```python
from build123d import *

# Parameters (mm, degrees)
SKETCH2_R               = 1
BOSS_EXTRUDE2_DEPTH     = 10
SKETCH4_R               = 3.5
BOSS_EXTRUDE3_DEPTH     = 10
CHAMFER1_SIZE           = 5.282754963
CHAMFER1_SIZE_2         = 3.05
CUT_EXTRUDE4_DEPTH      = 21.603397778
CUT_EXTRUDE4_DEPTH_BACK = 21.603397778
SKETCH5_R               = 1
SKETCH6_R               = 1.5
BOSS_EXTRUDE4_DEPTH     = 1
SKETCH7_R               = 2
BOSS_EXTRUDE5_DEPTH     = 4
CHAMFER2_SIZE           = 0.5


# Some blends are built 0.0001 mm under size
with BuildPart() as part:
    # Sketch1 → Revolve1 (revolve)
    with BuildSketch(Plane.XY):
        with BuildLine():
            Line((0, 0), (0, -2))
            ThreePointArc((0, -2), (2, 0), (0, 2))
            Line((0, 2), (0, 0))
        make_face()
    revolve(axis=Axis((0, 0, 0), (0, 1, 0)))

    # Sketch2 → Boss-Extrude2 (add)
    with BuildSketch(Plane(origin=(0, 0, 0), x_dir=(1, 0, 0), z_dir=(0, 1, 0))):
        with Locations(Location((0, 0, 0), (0, 0, 90))):
            Circle(SKETCH2_R)
    extrude(amount=BOSS_EXTRUDE2_DEPTH)

    # Sketch4 → Boss-Extrude3 (add)
    with BuildSketch(Plane(origin=(0, 10, 0), x_dir=(1, 0, 0), z_dir=(0, 1, 0))):
        with Locations(Location((0, 0, 0), (0, 0, 270))):
            Circle(SKETCH4_R)
    extrude(amount=BOSS_EXTRUDE3_DEPTH)

    # Chamfer1
    # the kernel refuses this chamfer: 5.282754963, 3.05 mm, written as the material it takes off along each edge
    with BuildSketch(Plane(origin=(0, 10, 0), x_dir=(0, 0, 1), z_dir=(-1, 0, 0))) as chamfer1_piece_1_section:
        Polygon((3.5, CHAMFER1_SIZE), (3.5 - CHAMFER1_SIZE_2, 0), (3.5, 0), align=None)
    chamfer1_piece_1 = revolve(axis=Axis((0, 10, 0), (0, 1, 0)), mode=Mode.PRIVATE)
    chamfer1_piece_1 = chamfer1_piece_1 - Plane(origin=(0, 13.183046822, 0), x_dir=(0, 0, -1), z_dir=(0, -1, 0)) * Cylinder(1, 22, mode=Mode.PRIVATE)
    add(chamfer1_piece_1, mode=Mode.SUBTRACT)

    # Sketch5 → Cut-Extrude4 (cut, two sides: drawn at the far end of the back side and taken through both)
    with BuildSketch(Plane(origin=(0, 0, 0), x_dir=(0, 0, -1), z_dir=(1, 0, 0)).offset(-CUT_EXTRUDE4_DEPTH_BACK)):
        with Locations((0, 17.641377482)):
            Circle(SKETCH5_R)
    extrude(amount=CUT_EXTRUDE4_DEPTH + CUT_EXTRUDE4_DEPTH_BACK, mode=Mode.SUBTRACT)

    # Sketch6 → Boss-Extrude4 (add)
    with BuildSketch(Plane(origin=(0, 20, 0), x_dir=(1, 0, 0), z_dir=(0, 1, 0))):
        with Locations(Location((0, 0, 0), (0, 0, 270))):
            Circle(SKETCH6_R)
    extrude(amount=BOSS_EXTRUDE4_DEPTH)

    # Sketch7 → Boss-Extrude5 (add)
    with BuildSketch(Plane(origin=(0, 21, 0), x_dir=(1, 0, 0), z_dir=(0, 1, 0))):
        with Locations(Location((0, 0, 0), (0, 0, 270))):
            Circle(SKETCH7_R)
    extrude(amount=BOSS_EXTRUDE5_DEPTH)

    # Chamfer2
    chamfer2_edges = [part.edges().sort_by_distance(p)[0] for p in [
        (0, 21, -2),
        (0, 25, -2),
    ]]
    chamfer(chamfer2_edges, length=CHAMFER2_SIZE - 0.0001)  # a hair under: the kernel refuses the full size


solid = part.part
```
Source: CAD feature listing. Evaluate the final solid. Frame: model axes, mm. A direction names the side the tool comes from. Give positions to 0.01 mm unless a question says otherwise; leave off trailing zeros. Order: outer loops, then holes, each group sorted by start corner. A loop starts at its lowest first (then second) coordinate and runs counter-clockwise, first axis right, second up.
(1) Contact query for flat-ended pins moving along their axis: P1, Ø2.5, axis at x = 0, z = -0.5, coming from the -Y side; P2, Ø3, axis at y = 15.5, z = 2, coming from the +X side; P3, Ø1, axis at y = 17, z = 1, coming from the -X side; P4, Ø2, axis at x = -1.5, y = 18, coming from the -Z side. Output: stop coordinate, or through.
(2) Section query D-D (y = 23.25). Return the cut outline in (x, z), plus the area to 3 significant figures.
(3) Material intervals for line 1 along Y through (x, z) = (1, 1.25); line 2 along Y through (x, z) = (-1.75, 0); line 3 along Y through (x, z) = (0.75, 1.5), sorted ascending.
(4) Access query for faces 1 (the face through (0, 20, 2)), 2 (the face through (-0.049, 16.754, -0.461)). Directions: +Z, -Z, +X, -X, +Y, -Y. A direction counts if a zero-diameter tool reaches every point of the face in a straight line with its end or side. Return the directions, or none.
(5) Pull-direction query (Y, two-part tool) for faces 3 (the face through (-1, 6, 0)), 4 (the face through (0, 25, 0)), 5 (the face through (-2, 23, 0)); classes: +Y half, -Y half, draft (parallel to the pull), parting line (faces both ways), or undercut.
(6) Section query B-B (x = 1.25). State how many separate pieces and enclosed holes the cut face has, plus the area to 3 significant figures.
Outcome:
1. P1: stops at y = -2
1. P2: stops at x = 3.46
1. P3: stops at x = -3.46
1. P4: stops at z = -3.46
2. outline: circle Ø4 at (0, 0)
2. area: 12.6 mm2
3. line 1: y = -1.2 to 1.2, 11.99 to 20, 21.1 to 24.9
3. line 2: y = -0.97 to 0.97, 12.25 to 16.64, 18.64 to 20, 21.25 to 24.75
3. line 3: y = -1.09 to 1.09, 12.13 to 20, 21.18 to 24.82
4. face 1: none
4. face 2: +X, -X
5. face 3: undercut
5. face 4: +Y half
5. face 5: draft
6. separate pieces: 2
6. enclosed holes: 1
6. area: 64.1 mm2
